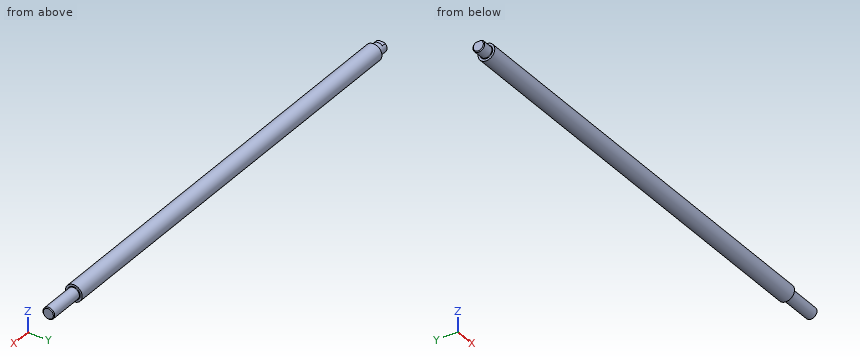
```python
from build123d import *

# Parameters (mm, degrees)
SKETCH1_W           = 258
SKETCH1_H           = 5
SKETCH2_R           = 3.5
BOSS_EXTRUDE1_DEPTH = 7
CUT_EXTRUDE1_START  = -3
CUT_EXTRUDE1_DEPTH  = 3
BOSS_EXTRUDE2_START = 22
SKETCH4_R           = 3.5
BOSS_EXTRUDE2_DEPTH = 22
CHAMFER1_SIZE       = 0.5
FILLET1_R           = 0.3


with BuildPart() as part:
    # Sketch1 → Revolve1 (revolve)
    with BuildSketch(Plane.XY, mode=Mode.PRIVATE) as revolve1_sk:
        with Locations((136, 2.5)):
            Rectangle(SKETCH1_W, SKETCH1_H)
    revolve(revolve1_sk.sketch.rotate(Axis((7, 0, 0), (1, 0, 0)), 270), axis=Axis((7, 0, 0), (1, 0, 0)))

    # Sketch2 → Boss-Extrude1 (add)
    with BuildSketch(Plane.ZY.offset(-7)):
        Circle(SKETCH2_R)
    extrude(amount=BOSS_EXTRUDE1_DEPTH)

    # Sketch3 → Cut-Extrude1 (cut)
    with BuildSketch(Plane.ZY.offset(CUT_EXTRUDE1_START)):
        with BuildLine():
            Line((2.5, 2.449489743), (2.5, -2.449489743))
            ThreePointArc((2.5, -2.449489743), (3.5, 0), (2.5, 2.449489743))
        make_face()
    extrude(amount=CUT_EXTRUDE1_DEPTH, mode=Mode.SUBTRACT)

    # Sketch4 → Boss-Extrude2 (add)
    with BuildSketch(Plane(origin=(265, 0, 0), x_dir=(0, 0, -1), z_dir=(1, 0, 0)).offset(BOSS_EXTRUDE2_START)):
        with Locations(Location((0, 0, 0), (0, 0, 135.584691403))):
            Circle(SKETCH4_R)
    extrude(amount=-BOSS_EXTRUDE2_DEPTH)

    # Chamfer1
    chamfer1_edges = [part.edges().sort_by_distance(p)[0] for p in [
        (287, -2.449489743, -2.5),
        (0, 0, -3.5),
    ]]
    chamfer(chamfer1_edges, length=CHAMFER1_SIZE)

    # Fillet1
    fillet1_edges = [part.edges().sort_by_distance(p)[0] for p in [
        (265, -2.449489743, -2.5),
        (7, 0, -3.5),
    ]]
    fillet(fillet1_edges, radius=FILLET1_R)


solid = part.part
```
Design review of the part built by this model. Coordinates are the model's own, in mm. Round coordinates to 2 decimals unless told otherwise and drop trailing zeros. Order: outer loops, then holes, each group sorted by start corner. A loop starts at its lowest first (then second) coordinate and runs counter-clockwise, first axis right, second up. Notation, with made-up numbers: (79.25, 29.25) - (132.25, 29.25) arc R24 cw to (132.25, 49.25) - close; hole circle Ø7 at (3.25, -33.75). An arc over 180 degrees is marked (long way). Return JSON: item names as keys, results as strings.
Q1. Consider section A-A on z = 0. Write out the cut boundary in (x, y), plus the area to 3 significant figures.
Computed values:
{"outline": "(0, -3) - (0.5, -3.5) - (6.7, -3.5) arc R0.3 cw to (7, -3.8) - (7, -5) - (265, -5) - (265, -3.8) arc R0.3 cw to (265.3, -3.5) - (286.5, -3.5) - (287, -3) - (287, 3) - (286.5, 3.5) - (265.3, 3.5) arc R0.3 cw to (265, 3.8) - (265, 5) - (7, 5) - (7, 3.8) arc R0.3 cw to (6.7, 3.5) - (0.5, 3.5) - (0, 3) - close", "area": "2,780 mm2"}
Q2. Wall thickness on L1, parallel to X at y = 3.75, z = 3; L2, parallel to Y at x = 96.5, z = 3.25; L3, parallel to Y at x = 141.5, z = -0.25: over which ranges is each line inside the solid? List them lowest first. Write a range as [from, to].
Computed values:
{"L1": "x = [7, 265]", "L2": "y = [-3.8, 3.8]", "L3": "y = [-4.99, 4.99]"}
Q3. Consider section B-B on x = 173. Write out the cut boundary in (y, z).
Computed values:
{"outline": "circle Ø10 at (0, 0)"}
Q4. For pin 1 Ø2.5 at (x, y) = (1, -0.5) entering from +Z; pin 2 Ø0.8 at (y, z) = (-1, 3) entering from -X; pin 3 Ø4 at (x, y) = (170.5, 2.5) entering from -Z, all flat-tipped, find the tip position at first contact; note any pin that passes through.
Computed values:
{"pin 1": "stops at z = 2.5", "pin 2": "stops at x = 3", "pin 3": "stops at z = -4.97"}
